from build123d import *

# Parameters (mm, degrees)
SALIENTE_EXTRUIR1_DEPTH = 5.75
CROQUIS3_R              = 3.175
SALIENTE_EXTRUIR2_DEPTH = 8.7
CROQUIS5_R              = 4.17
SALIENTE_EXTRUIR3_DEPTH = 9.4
CROQUIS6_R              = 1.11
CORTAR_EXTRUIR1_DEPTH   = 24.85
CHAFL_N1_SIZE           = 0.25


with BuildPart() as part:
    # Croquis2 → Saliente-Extruir1 (new body)
    with BuildSketch(Plane.XY):
        Polygon((4.859109949, 4.189463282), (-1.198626656, 6.302844296), (-6.057736605, 2.113381014), (-4.859109949, -4.189463282), (1.198626656, -6.302844296), (6.057736605, -2.113381014), align=None)
    extrude(amount=SALIENTE_EXTRUIR1_DEPTH)

    # Croquis3 → Saliente-Extruir2 (add)
    with BuildSketch(Plane.XY.offset(5.75)):
        Circle(CROQUIS3_R)
    extrude(amount=SALIENTE_EXTRUIR2_DEPTH)

    # Croquis5 → Saliente-Extruir3 (add)
    with BuildSketch(Plane(origin=(0, 0, 0), x_dir=(-1, 0, 0), z_dir=(0, 0, -1))):
        Circle(CROQUIS5_R)
    extrude(amount=SALIENTE_EXTRUIR3_DEPTH)

    # Croquis6 → Cortar-Extruir1 (cut, through all)
    with BuildSketch(Plane(origin=(0, 0, -9.4), x_dir=(-1, 0, 0), z_dir=(0, 0, -1))):
        Circle(CROQUIS6_R)
    extrude(amount=-CORTAR_EXTRUIR1_DEPTH, mode=Mode.SUBTRACT)

    # Chaflán1
    chafl_n1_edges = [part.edges().sort_by_distance(p)[0] for p in [
        (4.17, 0, 0),
        (4.17, 0, -9.4),
        (1.11, 0, -9.4),
    ]]
    chamfer(chafl_n1_edges, length=CHAFL_N1_SIZE)


solid = part.part
Could you check a few things on this model? Use its own coordinates, in mm. A direction names the side the tool comes from. Give positions to 0.01 mm unless a question says otherwise; leave off trailing zeros. Write each loop counter-clockwise with the first axis right and the second up, starting at its lowest first coordinate (ties: lowest second). Pieces come first, ordered by that corner, then holes. Notation, with made-up numbers: (-5.75, 48) -> (39.25, 48) arc R17 cw to (39.25, 81) -> close; hole circle Ø7 at (19, 58.25). An arc over 180 degrees is marked (long way). Answer as a JSON object with one key per item and string values.
Q1. Suppose I cut it at C-C on x = 0. Write out the boundary of the cut face in (y, z) (3 decimals).
Taken from the geometry:
{"outline": "(-5.885, 0) -> (-4.42, 0) -> (-4.17, -0.25) -> (-4.17, -9.15) -> (-3.92, -9.4) -> (-1.36, -9.4) -> (-1.11, -9.15) -> (-1.11, 14.45) -> (-3.175, 14.45) -> (-3.175, 5.75) -> (-5.885, 5.75) -> close; (1.11, -9.15) -> (1.36, -9.4) -> (3.92, -9.4) -> (4.17, -9.15) -> (4.17, -0.25) -> (4.42, 0) -> (5.885, 0) -> (5.885, 5.75) -> (3.175, 5.75) -> (3.175, 14.45) -> (1.11, 14.45) -> close"}
Q2. Please list where these lines run through material, in increasing order: L1, parallel to Y at x = 0, z = 7.5 (3 decimals); L2, parallel to Z at x = -3, y = 2.5; L3, parallel to Z at x = 3.75, y = 4.25.
Taken from the geometry:
{"L1": "y = -3.175 to -1.11, 1.11 to 3.175", "L2": "z = -9.4 to 5.75", "L3": "z = 0 to 5.75"}
Q3. Which directions (+Z, -Z, +X, -X, +Y, -Y) give clear straight access to the entire face, cutting with the end or side of a thin tool? Please do faces 4 (the cylindrical face through (-0.69, -3.1, 10.04)), 5 (the flat face through (-5.467, -0.994, 2.835)), 6 (the flat face through (4, -3, 0)).
Taken from the geometry:
{"face 4": "+Z", "face 5": "+Z, -Z, -X, -Y", "face 6": "-Z"}
Q4. Suppose I cut it at D-D on z = -5.5. Write out the boundary of the cut face in (x, y), then the cut area to 3 significant figures.
Taken from the geometry:
{"outline": "circle Ø8.34 at (0, 0); hole circle Ø2.22 at (0, 0)", "area": "50.8 mm²"}
Q5. Suppose I cut it at A-A on z = 5.25. Write out the boundary of the cut face in (x, y), then the cut area to 3 significant figures.
Taken from the geometry:
{"outline": "(-6.06, 2.11) -> (-4.86, -4.19) -> (1.2, -6.3) -> (6.06, -2.11) -> (4.86, 4.19) -> (-1.2, 6.3) -> close; hole circle Ø2.22 at (0, 0)", "area": "103 mm²"}
Q6. Suppose I cut it at B-B on y = 0. Write out the boundary of the cut face in (x, z) (3 decimals).
Taken from the geometry:
{"outline": "(-5.656, 0) -> (-4.42, 0) -> (-4.17, -0.25) -> (-4.17, -9.15) -> (-3.92, -9.4) -> (-1.36, -9.4) -> (-1.11, -9.15) -> (-1.11, 14.45) -> (-3.175, 14.45) -> (-3.175, 5.75) -> (-5.656, 5.75) -> close; (1.11, -9.15) -> (1.36, -9.4) -> (3.92, -9.4) -> (4.17, -9.15) -> (4.17, -0.25) -> (4.42, 0) -> (5.656, 0) -> (5.656, 5.75) -> (3.175, 5.75) -> (3.175, 14.45) -> (1.11, 14.45) -> close"}
Q7. Will these pins go through, and if not, where does the flat tip stop? pin 1 Ø1.5 at (x, z) = (0.5, -5.5) entering from -Y; pin 2 Ø5 at (y, z) = (1, -5) entering from -X; pin 3 Ø1.5 at (x, y) = (4.5, 5) entering from -Z.
Taken from the geometry:
{"pin 1": "stops at y = -4.17", "pin 2": "stops at x = -4.17", "pin 3": "stops at z = 0"}
Q8. We'd pull the mould along X, two halves only. Please class faces 1 (the flat face through (5.467, 0.994, 2.835)), 2 (the flat face through (3, 3, 5.75)), 3 (the cylindrical face through (0.241, -1.084, 2.485)): released by +X, released by -X, zero draft, split by the parting line, or undercut.
Taken from the geometry:
{"face 1": "released by +X", "face 2": "zero draft", "face 3": "undercut"}
